Work out the finished part from the listing and answer in its coordinate system (mm). Face numbers are marked on the shaded views. Coordinates: 2 decimals unless noted, no trailing zeros. Order: outer loops, then holes, each group sorted by start corner. A loop starts at its lowest first (then second) coordinate and runs counter-clockwise, first axis right, second up. Notation, with made-up numbers: (-5, -29.5) -> (27, -29.5) arc R29 ccw to (27, 7.5) -> close; hole circle Ø4 at (19.5, 25). An arc over 180 degrees is marked (long way). Write item = value, one per line. Start each with the question number.
Q1. The part is cut by section A-A, the plane z = 0.75. Count the separate pieces of the cut face and the enclosed holes in it, plus the area to 3 significant figures.
Q2. Flat-ended cylindrical pins translate along their axes: pin 1 (4 mm diameter, centred on x = 10.5, z = 6, fed in from -Y); pin 2 (3 mm diameter, centred on x = 2, z = 6, fed in from -Y); pin 3 (2.5 mm diameter, centred on x = 7, y = 7, fed in from -Z). Find the tip coordinate at first contact, or state that the pin passes through.
Q3. The part is cut by section D-D, the plane x = 12. Determine the outline of the cut face in (y, z).
Q4. The part is cut by section B-B, the plane x = 5.5. Determine the outline of the cut face in (y, z).
Q5. For a pull along Y with two mould halves and no side action, classify the marked faces 1, 2, 3 and 4 as +Y half, -Y half, draft (parallel to the pull), parting line (faces both ways), or undercut.
Q6. Straight lines are drawn through the part: L1, parallel to Y at x = 7, z = 6.75; L2, parallel to Y at x = 8.5, z = 7; L3, parallel to X at y = 55, z = 7.75. For each, find the intervals that lie inside material, in ascending order. Write a range as from..to.
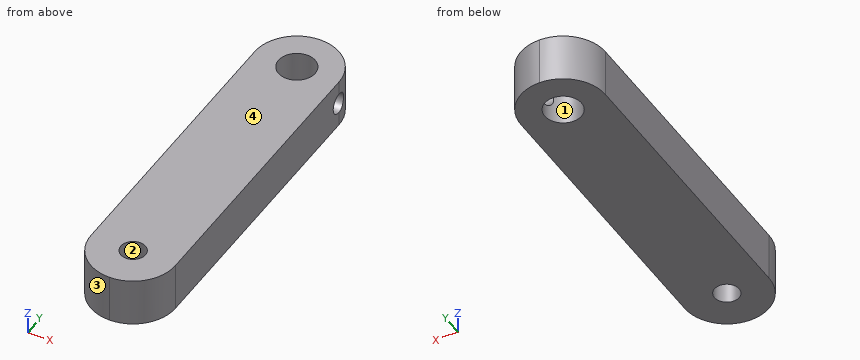
```python
from build123d import *

# Parameters (mm, degrees)
ESQUISSE2_W                  = 14
ESQUISSE2_H                  = 62
BOSS_EXTRU_1_DEPTH           = 8
ENL_V_MAT_EXTRU_1_DEPTH      = 65.062469512
ENL_V_MAT_EXTRU_1_DEPTH_BACK = 65.062469512
ESQUISSE3_R                  = 3.05
ESQUISSE3_R_2                = 2.05
CONG_1_R                     = 7
ENL_V_MAT_EXTRU_2_REACH      = 66.062
ENL_V_MAT_EXTRU_2_END_RADIUS = 3.05
ESQUISSE4_R                  = 1.7


with BuildPart() as part:
    # Esquisse2 → Boss.-Extru.1 (new body)
    with BuildSketch(Plane.XY):
        with Locations((7, 31)):
            Rectangle(ESQUISSE2_W, ESQUISSE2_H)
    extrude(amount=BOSS_EXTRU_1_DEPTH)

    # Esquisse3 → Enlèv. mat.-Extru.1 (cut, two sides: drawn at the far end of the back side and taken through both)
    with BuildSketch(Plane.XY.offset(8).offset(-ENL_V_MAT_EXTRU_1_DEPTH_BACK)):
        with Locations((7, 55)):
            Circle(ESQUISSE3_R)
        with Locations(Location((7, 7, 0), (0, 0, 180))):
            Circle(ESQUISSE3_R_2)
    extrude(amount=ENL_V_MAT_EXTRU_1_DEPTH + ENL_V_MAT_EXTRU_1_DEPTH_BACK, mode=Mode.SUBTRACT)

    # Congé1
    cong_1_edges = [part.edges().sort_by_distance(p)[0] for p in [
        (14, 0, 4),
        (0, 0, 4),
        (0, 62, 4),
        (14, 62, 4),
    ]]
    fillet(cong_1_edges, radius=CONG_1_R - 0.0001)  # a hair under: the kernel refuses the full size

    # Enlèv. mat.-Extru.2: up to this cylinder (the profile starts outside it)
    enl_v_mat_extru_2_end = Plane(origin=(7, 55, 4), z_dir=(0, 0, 1)) * Cylinder(ENL_V_MAT_EXTRU_2_END_RADIUS, 139.224, mode=Mode.PRIVATE)
    # Esquisse4 → Enlèv. mat.-Extru.2 (cut, up to the surface)
    with BuildSketch(Plane(origin=(14, 0, 0), x_dir=(0, 0, -1), z_dir=(1, 0, 0)), mode=Mode.PRIVATE) as enl_v_mat_extru_2_sk1:
        with Locations((-4, 55)):
            Circle(ESQUISSE4_R)
    enl_v_mat_extru_2_tool1 = extrude(enl_v_mat_extru_2_sk1.sketch, amount=-ENL_V_MAT_EXTRU_2_REACH, mode=Mode.PRIVATE) - enl_v_mat_extru_2_end
    add(enl_v_mat_extru_2_tool1.solids().sort_by_distance((14, 55, 4))[0], mode=Mode.SUBTRACT)


solid = part.part
```
Model answer:
q1.separate_pieces = 1
q1.enclosed_holes = 2
q1.area = 784 mm2
q2.pin_1 = 0.16
q2.pin_2 = 0.94
q2.pin_3 = through
q3.outline = (2.1, 0) -> (59.9, 0) -> (59.9, 8) -> (2.1, 8) -> close; hole circle Ø3.4 at (55, 4)
q4.outline = (0.16, 0) -> (5.6, 0) -> (5.6, 8) -> (0.16, 8) -> close; (8.4, 0) -> (52.34, 0) -> (52.34, 8) -> (8.4, 8) -> close; (57.66, 0) -> (61.84, 0) -> (61.84, 8) -> (57.66, 8) -> close
q5.face_1 = undercut
q5.face_2 = undercut
q5.face_3 = -Y half
q5.face_4 = draft
q6.L1 = 0..4.95, 9.05..51.95, 58.05..62
q6.L2 = 0.16..5.6, 8.4..52.34, 57.66..61.84
q6.L3 = 0..3.95, 10.05..14
